from build123d import *

# Parameters (mm, degrees)
F0_R             = 22.225
F0_R_2           = 2.15265
F1_DEPTH         = 9.525
F3_DEPTH         = 9.525
F4_COUNT         = 6
F4_ANGLE         = 300
F6_R             = 11.90625
F7_DEPTH         = 8.29945
F10_R            = 3.96875
F11_DEPTH        = 6.35
F12_R            = 3.96875
F13_DEPTH        = 6.35
F15_DEPTH        = 9.525
F15_COPIES_COUNT = 4


# Not quite as in the source:
# - a pattern or mirror of a feature is missing from the dataset's text; its kind, count and spacing are read off the source's solid


with BuildPart() as f1:
    # F0 (on Top) → F1 (new body)
    with BuildSketch(Plane.XY):
        Circle(F0_R)
        with Locations((-11.7865861589, -11.7865861589)):
            Circle(F0_R_2, mode=Mode.SUBTRACT)
        with Locations((11.7865861589, -11.7865861589)):
            Circle(F0_R_2, mode=Mode.SUBTRACT)
        with Locations((-11.7865861589, 11.7865861589)):
            Circle(F0_R_2, mode=Mode.SUBTRACT)
        with BuildLine():
            ThreePointArc((0, 11.1125), (7.8577241059, 7.8577241059), (11.1125, 0))
            ThreePointArc((11.1125, 0), (-7.8577241059, -7.8577241059), (0, 11.1125))
        make_face(mode=Mode.SUBTRACT)
        with Locations((11.7865861589, 11.7865861589)):
            Circle(F0_R_2, mode=Mode.SUBTRACT)
    extrude(amount=F1_DEPTH)

    # F2 (on face) → F3 (cut, through all)
    with BuildSketch(Plane.XY.offset(9.525)):
        with BuildLine():
            ThreePointArc((-2.8761266387, 10.7338507446), (0, 11.1125), (2.8761266387, 10.7338507446))
            Line((2.8761266387, 10.7338507446), (3.0815642558, 11.5005543693))
            ThreePointArc((3.0815642558, 11.5005543693), (0, 11.90625), (-3.0815642558, 11.5005543693))
            Line((-3.0815642558, 11.5005543693), (-2.8761266387, 10.7338507446))
        make_face()
    f3 = extrude(amount=-F3_DEPTH, mode=Mode.SUBTRACT)

    # F4: F3 ×6 about axis
    f4_axis = Axis((0, 0, 0), (0, 0, -1))
    for i in range(1, F4_COUNT):
        add(f3.rotate(f4_axis, i * F4_ANGLE / (F4_COUNT - 1)), mode=Mode.SUBTRACT)

    # F6 (on face) → F7 (cut, through all)
    with BuildSketch(Plane(origin=(0, 0, 0), x_dir=(1, 0, 0), z_dir=(0, 0, -1))):
        Circle(F6_R)
    extrude(amount=-F7_DEPTH, mode=Mode.SUBTRACT)

    # F10 (on face) → F11 (cut, through all)
    with BuildSketch(Plane(origin=(0, 0, 0), x_dir=(1, 0, 0), z_dir=(0, 0, -1))):
        with Locations((11.7865861589, -11.7865861589)):
            Circle(F10_R)
        with Locations((-11.7865861589, 11.7865861589)):
            Circle(F10_R)
    extrude(amount=-F11_DEPTH, mode=Mode.SUBTRACT)

    # F12 (on face) → F13 (cut, through all)
    with BuildSketch(Plane.XY.offset(9.525)):
        with Locations((-11.7865861589, 11.7865861589)):
            Circle(F12_R)
        with Locations((11.7865861589, -11.7865861589)):
            Circle(F12_R)
    extrude(amount=-F13_DEPTH, mode=Mode.SUBTRACT)

    # F14 (on face) → F15 (cut, through all)
    with BuildSketch(Plane(origin=(0, 0, 0), x_dir=(1, 0, 0), z_dir=(0, 0, -1))):
        with BuildLine():
            ThreePointArc((-11.229543123, 17.3148424047), (-8.3361072587, 16.1415958514), (-6.5322351826, 13.5931602316))
            ThreePointArc((-6.5322351826, 13.5931602316), (0, 15.08125), (6.5322351826, 13.5931602316))
            ThreePointArc((6.5322351826, 13.5931602316), (8.3361072587, 16.1415958514), (11.229543123, 17.3148424047))
            ThreePointArc((11.229543123, 17.3148424047), (0, 20.6375), (-11.229543123, 17.3148424047))
        make_face()
    f15 = extrude(amount=-F15_DEPTH, mode=Mode.SUBTRACT)

    # F15_copies: F15 ×4 about axis
    f15_copies_axis = Axis((0, 0, 0), (0, 0, 1))
    for i in range(1, F15_COPIES_COUNT):
        add(f15.rotate(f15_copies_axis, i * 360 / F15_COPIES_COUNT), mode=Mode.SUBTRACT)


solid = f1.part
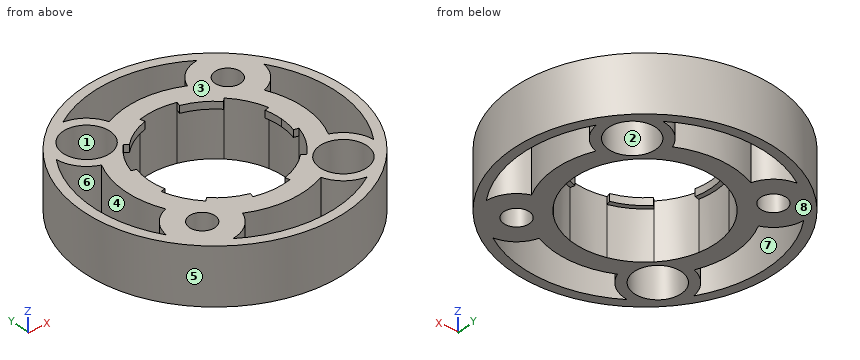
For this review, take the finished solid that the model builds, in its own axes (mm). Face numbers are marked on the shaded views. A direction names the side the tool comes from. Round coordinates to 2 decimals unless told otherwise and drop trailing zeros. Loops run counter-clockwise (first coordinate to the right, second up) from the corner with the lowest first, then second, coordinate; pieces in that order, holes last. Notation, with made-up numbers: (-9.5, 48) - (9.5, 48) arc R10 ccw to (9.5, 52) - close; hole circle Ø3 at (21.5, 2). An arc over 180 degrees is marked (long way). Put each result on its own line as item: value. Start each with the question number.
1. Consider section A-A on x = 0. State the section outline as (y, z) points (1 decimal).
2. Mouldability with a two-part tool opening along X and no side actions: class the marked faces 5, 6, 7 and 8 as +X half, -X half, draft (parallel to the pull), parting line (faces both ways), or undercut.
3. For probe 1 along X at (y, z) = (2.5, 1); probe 2 along X at (y, z) = (13, 0.75); probe 3 along X at (y, z) = (5, 8), list the stretches that pass through material, from the lowest coordinate up. Write a range as [from, to].
4. Consider section D-D on y = -19. State the section outline as (x, z) points (3 decimals).
5. Insertion check: P1, Ø9, axis at x = 11.79, y = -11.79, coming from the -Z side; P2, Ø7, axis at x = 11.79, y = 11.79, coming from the -Z side; P3, Ø7, axis at x = 11.79, y = -11.79, coming from the +Z side (3 decimals); P4, Ø1, axis at x = 10.5, z = 2.5, coming from the -Y side. Each pin has a flat end and moves straight along its axis. Give the tip position at first contact, or say it passes through.
6. Consider section B-B on y = -13. State the section outline as (x, z) points (3 decimals).
7. For the marked faces 1, 2, 3 and 4, list the 3-axis set-ups (+Z, -Z, +X, -X, +Y, -Y) from which the entire face can be reached by the end or side of a thin tool; tool diameter is ignored.
8. Consider section C-C on z = 4.5. State how many separate pieces and enclosed holes the cut face has, plus the area to 3 significant figures.
Result sheet:
1. outline: (-22.2, 0) - (-20.6, 0) - (-20.6, 9.5) - (-22.2, 9.5) - close; (-15.1, 0) - (-11.9, 0) - (-11.9, 9.5) - (-15.1, 9.5) - close; (11.9, 0) - (15.1, 0) - (15.1, 9.5) - (11.9, 9.5) - close; (20.6, 0) - (22.2, 0) - (22.2, 9.5) - (20.6, 9.5) - close
2. face 5: parting line
2. face 6: undercut
2. face 7: undercut
2. face 8: draft
3. probe 1: [-22.08, -20.49], [-14.87, -11.64], [11.64, 14.87], [20.49, 22.08]
3. probe 2: [-18.03, -13.56], [-10.01, 8.01], [15.57, 18.03]
3. probe 3: [-21.66, -20.02], [-14.23, -10.81], [10.81, 14.23], [20.02, 21.66]
4. outline: (-11.53, 0) - (-8.056, 0) - (-8.056, 9.525) - (-11.53, 9.525) - close; (8.056, 0) - (11.53, 0) - (11.53, 9.525) - (8.056, 9.525) - close
5. P1: z = 0
5. P2: z = 6.35
5. P3: z = 3.175
5. P4: y = -19.85
6. outline: (-18.026, 0) - (-15.565, 0) - (-15.565, 6.35) - (-13.565, 6.35) - (-13.565, 9.525) - (-18.026, 9.525) - close; (-10.009, 6.35) - (-8.008, 6.35) - (-8.008, 0) - (10.009, 0) - (10.009, 3.175) - (8.008, 3.175) - (8.008, 9.525) - (-10.009, 9.525) - close; (13.565, 0) - (18.026, 0) - (18.026, 9.525) - (15.565, 9.525) - (15.565, 3.175) - (13.565, 3.175) - close
7. face 1: +Z
7. face 2: -Z
7. face 3: +Z, +X, -X, +Y, -Y
7. face 4: +Z, -Z
8. separate pieces: 1
8. enclosed holes: 9
8. area: 523 mm^2
